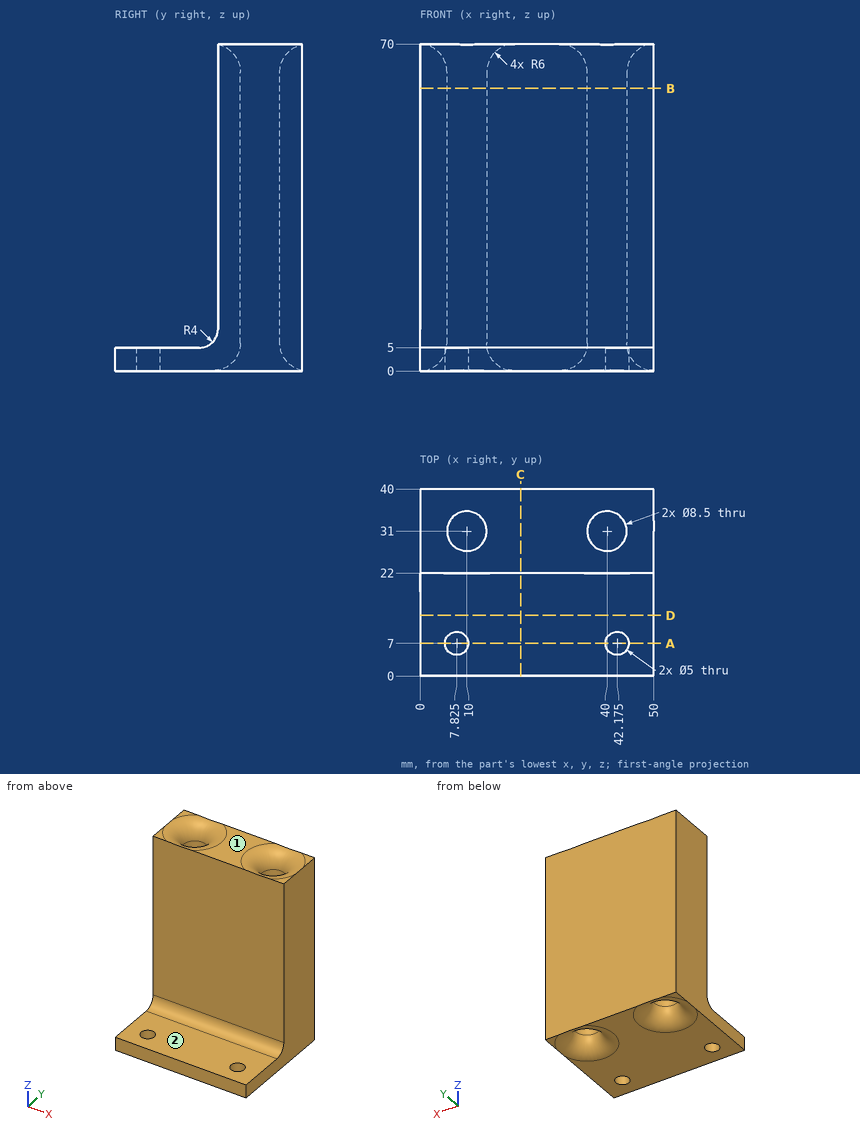
For this review, use the dimensioned drawing (mm, ordinates from the lowest corner) and the shaded views. A direction names the side the tool comes from. Coordinates: 2 decimals unless noted, no trailing zeros. Write each loop counter-clockwise with the first axis right and the second up, starting at its lowest first coordinate (ties: lowest second). Pieces come first, ordered by that corner, then holes. Notation, with made-up numbers: (40, 68.5) - (62, 68.5) arc R7 ccw to (62, 72.5) - close; hole circle Ø5 at (60.25, -34). An arc over 180 degrees is marked (long way). Answer in a Markdown table with one row per item. Add a question column.
Q1. Consider section D-D on y = 13. Give the boundary of the cut face in (x, z), then the cut area to 3 significant figures.
Q2. Consider section A-A on y = 7. Give the boundary of the cut face in (x, z) (3 decimals), then the cut area to 3 significant figures.
Q3. Consider section C-C on x = 21.5. Give the boundary of the cut face in (y, z).
Q4. Consider section B-B on z = 60.5. Give the boundary of the cut face in (x, y), then the cut area to 3 significant figures.
Q5. Clearance check with flat-ended pins moving along their axes: pin 1 (3 mm diameter, centred on x = 22.5, y = 18.5, fed in from +Z); pin 2 (15 mm diameter, centred on x = 34.5, z = 34.5, fed in from -Y); pin 3 (13.5 mm diameter, centred on x = 40, y = 31, fed in from +Z); pin 4 (4.5 mm diameter, centred on x = 7.825, y = 7, fed in from +Z). State where each tip first meets the part, or that it passes through.
Q6. For the marked faces 1 and 2, list the 3-axis set-ups (+Z, -Z, +X, -X, +Y, -Y) from which the entire face can be reached by the end or side of a thin tool; tool diameter is ignored.
Q7. To check wall thickness, follow line 1 along Y through (x, z) = (40, 48.5); line 2 along X through (y, z) = (27.5, 49); line 3 along X through (y, z) = (29.5, 58.5). State the ranges of each line that lie inside material, in increasing order. Write a range as from..to.
Answers below:
| question | item | result |
|---|---|---|
| 1 | outline | (0, 0) - (50, 0) - (50, 5) - (0, 5) - close |
| 1 | area | 250 mm² |
| 2 | outline | (0, 0) - (5.325, 0) - (5.325, 5) - (0, 5) - close; (10.325, 0) - (39.675, 0) - (39.675, 5) - (10.325, 5) - close; (44.675, 0) - (50, 0) - (50, 5) - (44.675, 5) - close |
| 2 | area | 200 mm² |
| 3 | outline | (0, 0) - (40, 0) - (40, 70) - (22, 70) - (22, 9) arc R4 cw to (18, 5) - (0, 5) - close |
| 4 | outline | (0, 22) - (50, 22) - (50, 40) - (0, 40) - close; hole circle Ø8.5 at (10, 31); hole circle Ø8.5 at (40, 31) |
| 4 | area | 787 mm² |
| 5 | pin 1 | z = 5.54 |
| 5 | pin 2 | y = 22 |
| 5 | pin 3 | z = 68.87 |
| 5 | pin 4 | through |
| 6 | face 1 | +Z, +X, -X, +Y, -Y |
| 6 | face 2 | +Z, +X, -X, -Y |
| 7 | line 1 | 22..26.75, 35.25..40 |
| 7 | line 2 | 0..7.59, 12.41..37.59, 42.41..50 |
| 7 | line 3 | 0..6.02, 13.98..36.02, 43.98..50 |
